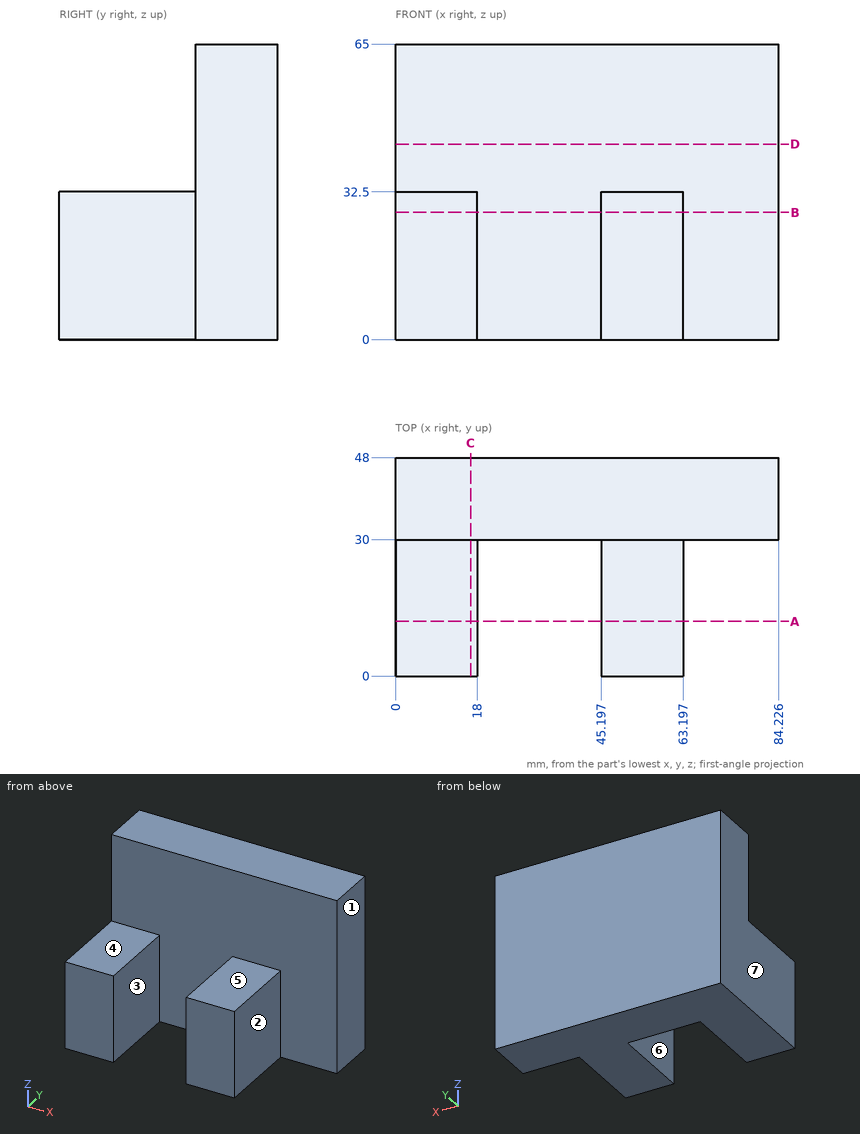
For this review, use the dimensioned drawing (mm, ordinates from the lowest corner) and the shaded views. A direction names the side the tool comes from. Coordinates: 2 decimals unless noted, no trailing zeros. Write each loop counter-clockwise with the first axis right and the second up, starting at its lowest first coordinate (ties: lowest second). Pieces come first, ordered by that corner, then holes. Notation, with made-up numbers: (1.25, 7) - (16.25, 7) arc R21 ccw to (16.25, 37) - close; hole circle Ø1 at (-4.5, 29). An arc over 180 degrees is marked (long way). Answer in a Markdown table with one row per item. Add a question column.
Q1. Consider section A-A on y = 12. Give the boundary of the cut face in (x, z), then the cut area to 3 significant figures.
Q2. Consider section C-C on x = 16.5. Give the boundary of the cut face in (y, z), then the cut area to 4 significant figures.
Q3. To check wall thickness, follow line 1 along X through (y, z) = (10.5, 21); line 2 along Z through (x, y) = (10.5, 8.5); line 3 along Y through (x, z) = (61, 54). State the ranges of each line that lie inside material, in increasing order. Write a range as from..to.
Q4. Consider section B-B on z = 28. Give the boundary of the cut face in (x, y), then the cut area to 3 significant figures.
Q5. Consider section D-D on z = 43. Give the boundary of the cut face in (x, y).
Q6. For the marked faces 1, 2, 3 and 4, list the 3-axis set-ups (+Z, -Z, +X, -X, +Y, -Y) from which the entire face can be reached by the end or side of a thin tool; tool diameter is ignored.
Q7. Draft analysis for pull direction X (two halves, no side actions). For the marked faces 5, 6 and 7, state which applies: +X half, -X half, draft (parallel to the pull), parting line (faces both ways), or undercut.
Q8. Clearance check with flat-ended pins moving along their axes: pin 1 (20 mm diameter, centred on x = 11.5, y = 14, fed in from +Z); pin 2 (9 mm diameter, centred on y = 8, z = 17.5, fed in from +X); pin 3 (12 mm diameter, centred on x = 74.5, z = 20, fed in from -Y). State where each tip first meets the part, or that it passes through.
Answers below:
| question | item | result |
|---|---|---|
| 1 | outline | (0, 0) - (18, 0) - (18, 32.5) - (0, 32.5) - close; (45.2, 0) - (63.2, 0) - (63.2, 32.5) - (45.2, 32.5) - close |
| 1 | area | 1,170 mm² |
| 2 | outline | (0, 0) - (48, 0) - (48, 65) - (30, 65) - (30, 32.5) - (0, 32.5) - close |
| 2 | area | 2,145 mm² |
| 3 | line 1 | 0..18, 45.2..63.2 |
| 3 | line 2 | 0..32.5 |
| 3 | line 3 | 30..48 |
| 4 | outline | (0, 0) - (18, 0) - (18, 30) - (45.2, 30) - (45.2, 0) - (63.2, 0) - (63.2, 30) - (84.23, 30) - (84.23, 48) - (0, 48) - close |
| 4 | area | 2,600 mm² |
| 5 | outline | (0, 30) - (84.23, 30) - (84.23, 48) - (0, 48) - close |
| 6 | face 1 | +Z, -Z, +X, +Y, -Y |
| 6 | face 2 | +Z, -Z, +X, -Y |
| 6 | face 3 | +Z, -Z, -Y |
| 6 | face 4 | +Z, +X, -X, -Y |
| 7 | face 5 | draft |
| 7 | face 6 | undercut |
| 7 | face 7 | -X half |
| 8 | pin 1 | z = 32.5 |
| 8 | pin 2 | x = 63.2 |
| 8 | pin 3 | y = 30 |
